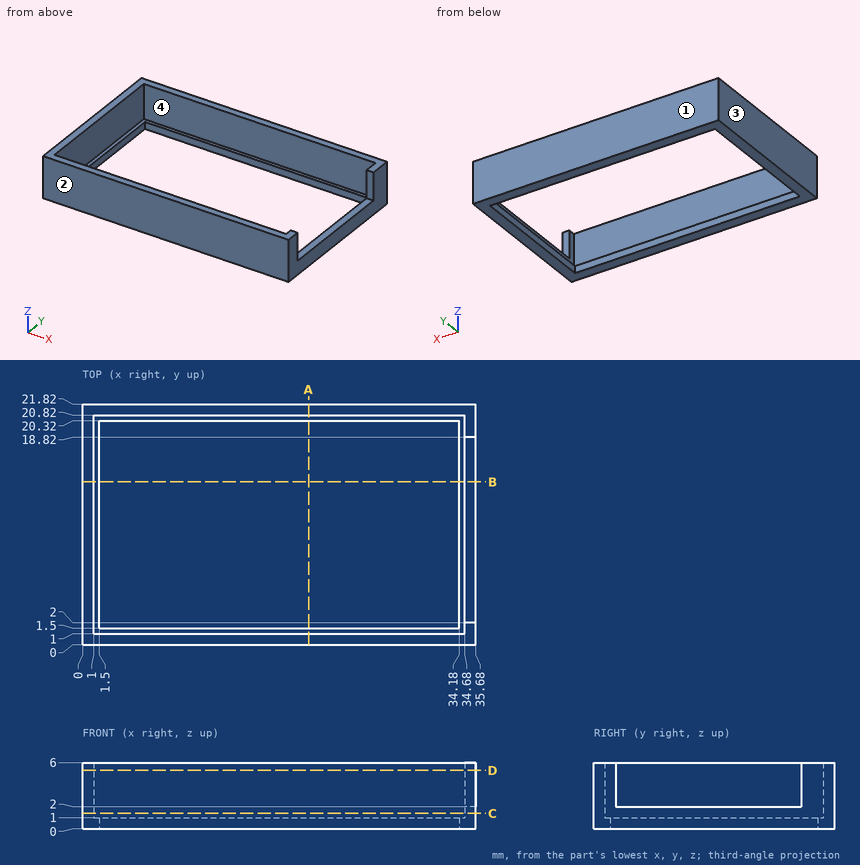
Could you check a few things on this drawing? It's one solid part, dimensions in mm from its lowest x, y, z. Coordinates: 2 decimals unless noted, no trailing zeros. Order: outer loops, then holes, each group sorted by start corner. A loop starts at its lowest first (then second) coordinate and runs counter-clockwise, first axis right, second up. Notation, with made-up numbers: M 15,22 L 29,22 A20 cw 29,35 Z; hole C 18,-2 d4. An arc over 180 degrees is marked long. Use one line per item in the form item = value. Start each with the question number.
1. Suppose I cut it at C-C on z = 1.4. Write out the boundary of the cut face in (x, y).
2. Suppose I cut it at B-B on y = 14.75. Write out the boundary of the cut face in (x, z), then the cut area to 3 significant figures.
3. We'd pull the mould along Y, two halves only. Please class the marked faces 1, 2, 3 and 4: +Y half, -Y half, draft (parallel to the pull), parting line (faces both ways), or undercut.
4. Suppose I cut it at A-A on x = 20.5. Write out the boundary of the cut face in (y, z).
5. Suppose I cut it at D-D on z = 5.3. Write out the boundary of the cut face in (x, y).
6. Please list where these lines run through material, in increasing order: line 1 (Y direction, x = 31, z = 1.2); line 2 (X direction, y = 11.5, z = 0.6); line 3 (Y direction, x = 3, z = 0.9).
7. For pin 1 (3 mm diameter, centred on x = 21.5, y = 4, fed in from -Z); pin 2 (1.1 mm diameter, centred on x = 35, y = 7.5, fed in from +Z), each with a flat end and sliding along its axis, tell me the tip position at first contact or that it passes through.
Geometry says:
q1.outline = M 0,0 L 35.68,0 L 35.68,21.82 L 0,21.82 Z; hole M 1,1 L 34.68,1 L 34.68,20.82 L 1,20.82 Z
q2.outline = M 0,0 L 1.5,0 L 1.5,1 L 1,1 L 1,6 L 0,6 Z; M 34.18,0 L 35.68,0 L 35.68,2 L 34.68,2 L 34.68,1 L 34.18,1 Z
q2.area = 9.00 mm^2
q3.face_1 = +Y half
q3.face_2 = -Y half
q3.face_3 = draft
q3.face_4 = undercut
q4.outline = M 0,0 L 1.5,0 L 1.5,1 L 1,1 L 1,6 L 0,6 Z; M 20.32,0 L 21.82,0 L 21.82,6 L 20.82,6 L 20.82,1 L 20.32,1 Z
q5.outline = M 0,0 L 35.68,0 L 35.68,2 L 34.68,2 L 34.68,1 L 1,1 L 1,20.82 L 34.68,20.82 L 34.68,18.82 L 35.68,18.82 L 35.68,21.82 L 0,21.82 Z
q6.line_1 = 0 to 1, 20.82 to 21.82
q6.line_2 = 0 to 1.5, 34.18 to 35.68
q6.line_3 = 0 to 1.5, 20.32 to 21.82
q7.pin_1 = through
q7.pin_2 = 2
